Verification items for the finished model (mm, model axes). Face numbers are marked on the shaded views. A direction names the side the tool comes from. Round coordinates to 2 decimals unless told otherwise and drop trailing zeros. Write each loop counter-clockwise with the first axis right and the second up, starting at its lowest first coordinate (ties: lowest second). Pieces come first, ordered by that corner, then holes. Notation, with made-up numbers: (84, 35) -> (92, 35) arc R15 ccw to (92, 49) -> close; hole circle Ø9 at (1, 48). An arc over 180 degrees is marked (long way). Use CSV: the item, a comma, the result in double quotes.
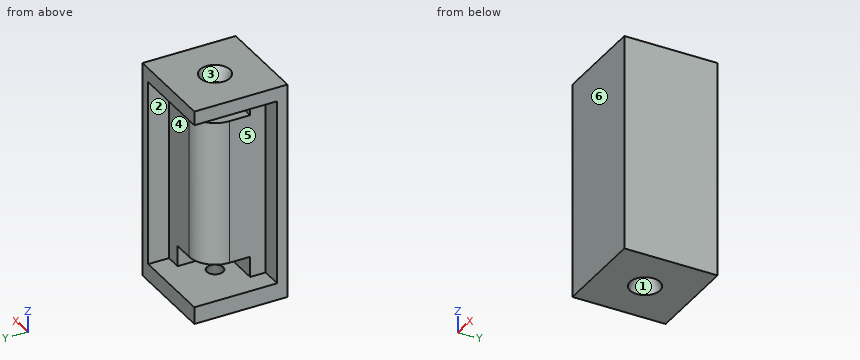
```python
from build123d import *

# Parameters (mm, degrees)
BOX013_W          = 18
BOX013_H          = 18
BOX013_DEPTH      = 36
CYLINDER006_R     = 1
CYLINDER006_DEPTH = 70
BOX011_W          = 18
BOX011_H          = 18
BOX011_DEPTH      = 4
ARRAY005_Z_COUNT  = 2
ARRAY005_Z_PITCH  = 32
BOX012_W          = 18
BOX012_H          = 18
BOX012_DEPTH      = 36
BOX010_W          = 18
BOX010_H          = 18
BOX010_DEPTH      = 42
FILLET_R          = 5


with BuildPart() as cube013:
    # Box013 → Box013 (new body)
    with BuildSketch(Plane(origin=(-2, 14, 3.3), x_dir=(1, 0, 0), z_dir=(0, 0, 1))):
        with Locations((9, 9)):
            Rectangle(BOX013_W, BOX013_H)
    extrude(amount=BOX013_DEPTH)


with BuildPart() as cylinder006:
    # Cylinder006 → Cylinder006 (new body)
    with BuildSketch(Plane(origin=(9, 9, -17), x_dir=(1, 0, 0), z_dir=(0, 0, 1))):
        Circle(CYLINDER006_R)
    extrude(amount=CYLINDER006_DEPTH)


with BuildPart() as array005:
    # Box011 → Box011 (new body)
    with BuildSketch(Plane(origin=(-5, 5, 3.3), x_dir=(1, 0, 0), z_dir=(0, 0, 1))):
        with Locations((9, 9)):
            Rectangle(BOX011_W, BOX011_H)
    extrude(amount=BOX011_DEPTH)

    # Array005 Z: Array005 ×2


with BuildPart() as array005_1:
    add(array005.part)
    with Locations(*[(0, 0, i * ARRAY005_Z_PITCH) for i in range(1, ARRAY005_Z_COUNT)]):
        add(array005.part)


with BuildPart() as cone:
    # Cone → Cone (revolve)
    with BuildSketch(Plane(origin=(9, 9, 0), x_dir=(1, 0, 0), z_dir=(0, -1, 0))):
        Polygon((0, 0), (2.9, 0), (1.5, 3.5), (0, 3.5), align=None)
    revolve(axis=Axis((9, 9, 0), (0, 0, 1)))


with BuildPart() as cone001:
    # Cone001 → Cone001 (revolve)
    with BuildSketch(Plane(origin=(9, 9, 38.5), x_dir=(1, 0, 0), z_dir=(0, -1, 0))):
        Polygon((0, 0), (1.5, 0), (2.9, 3.5), (0, 3.5), align=None)
    revolve(axis=Axis((9, 9, 38.5), (0, 0, 1)))


with BuildPart() as fusion003:
    # Box012 → Box012 (new body)
    with BuildSketch(Plane(origin=(-14, 2, 3.3), x_dir=(1, 0, 0), z_dir=(0, 0, 1))):
        with Locations((9, 9)):
            Rectangle(BOX012_W, BOX012_H)
    extrude(amount=BOX012_DEPTH)

    # Fusion003: union Cube013, Cylinder006, Array005, Cone, Cone001
    add(cube013.part)
    add(cylinder006.part)
    add(array005_1.part)
    add(cone.part)
    add(cone001.part)


with BuildPart() as corner_clone:
    # Box010 → Box010 (new body)
    with BuildSketch(Plane.XY):
        with Locations((9, 9)):
            Rectangle(BOX010_W, BOX010_H)
    extrude(amount=BOX010_DEPTH)

    # Cut005: cut Fusion003
    add(fusion003.part, mode=Mode.SUBTRACT)

    # Fillet
    fillet_edges = [corner_clone.edges().sort_by_distance(p)[0] for p in [
        (4, 14, 21.3),
    ]]
    fillet(fillet_edges, radius=FILLET_R)


solid = corner_clone.part
```
Q1. Section check B-B (x = 3.5). Record the cut outline in (y, z), plus the area to 3 significant figures.
Filled in:
outline,"(0, 0) -> (18, 0) -> (18, 3.3) -> (2, 3.3) -> (2, 39.3) -> (18, 39.3) -> (18, 42) -> (0, 42) -> close"
area,"180 mm²"
Q2. Section check A-A (z = 11). Record the cut outline in (x, y), plus the area to 3 significant figures.
Filled in:
outline,"(0, 0) -> (18, 0) -> (18, 18) -> (16, 18) -> (16, 14) -> (9, 14) arc R5 ccw to (4, 9) -> (4, 2) -> (0, 2) -> close; hole circle Ø2 at (9, 9)"
area,"203 mm²"
Q3. Section check C-C (y = 16.25). Record the cut outline in (x, z).
Filled in:
outline,"(0, 0) -> (18, 0) -> (18, 42) -> (0, 42) -> (0, 39.3) -> (16, 39.3) -> (16, 3.3) -> (0, 3.3) -> close"
Q4. Mould release check, pull along Y, two halves, no side actions. Record for the marked faces 1, 2, 3 and 4: released by +Y, released by -Y, zero draft, split by the parting line, or undercut.
Filled in:
face 1,"undercut"
face 2,"zero draft"
face 3,"undercut"
face 4,"released by +Y"
Q5. Section check D-D (z = 6). Record the cut outline in (x, y), plus the area to 3 significant figures.
Filled in:
outline,"(0, 0) -> (18, 0) -> (18, 18) -> (16, 18) -> (16, 14) -> (13, 14) -> (13, 5) -> (4, 5) -> (4, 2) -> (0, 2) -> close"
area,"131 mm²"
Q6. Access from +Z, -Z, +X, -X, +Y, -Y to the whole of each face (thin tool, end or side, straight path). Record for the marked faces 5 and 6.
Filled in:
face 5,"-X, +Y"
face 6,"+Z, -Z, +X, -X, -Y"
Q7. Go/stop test with flat-tipped pins: P1, Ø1.2, axis at y = 15.5, z = 12.5, coming from the -X side; P2, Ø8, axis at x = 6.5, z = 29.5, coming from the +Y side; P3, Ø2, axis at y = 7.5, z = 5.5, coming from the -X side. Record where each tip stops, or that it passes through.
Filled in:
P1,"x = 16"
P2,"y = 14"
P3,"x = 13"
Q8. Material ranges on L1, parallel to Z at x = 6.75, y = 12; L2, parallel to Z at x = 9.5, y = 16.75; L3, parallel to Y at x = 9, z = 16.75, recorded low to high.
Filled in:
L1,"0 to 3.3, 7.3 to 35.3, 39.3 to 42"
L2,"0 to 3.3, 39.3 to 42"
L3,"0 to 8, 10 to 14"
